```python
from build123d import *

# Parameters (mm, degrees)
F0_R     = 5
F1_DEPTH = 20
F2_R     = 1.25
F3_DEPTH = 20.001
F5_DEPTH = 10


with BuildPart() as f1:
    # F0 (on Front) → F1 (new body)
    with BuildSketch(Plane.XZ):
        Circle(F0_R)
    extrude(amount=F1_DEPTH)

    # F2 (on face) → F3 (cut, through all)
    with BuildSketch(Plane(origin=(0, 0, 0), x_dir=(-1, 0, 0), z_dir=(0, 1, 0))):
        Circle(F2_R)
    extrude(amount=-F3_DEPTH, mode=Mode.SUBTRACT)

    # F4 (on Front) → F5 (cut)
    with BuildSketch(Plane.XZ):
        Polygon((1.674316, 2.9), (-1.674316, 2.9), (-3.348632, 0), (-1.674316, -2.9), (1.674316, -2.9), (3.348632, 0), align=None)
    extrude(amount=F5_DEPTH, mode=Mode.SUBTRACT)


solid = f1.part
```
Can you work these out from the model? Positions are in its coordinate system, mm. A direction names the side the tool comes from. Round coordinates to 2 decimals unless told otherwise and drop trailing zeros. Loops run counter-clockwise (first coordinate to the right, second up) from the corner with the lowest first, then second, coordinate; pieces in that order, holes last.
Item 1: Suppose I cut it at B-B, the plane y = -8.75. Write out the boundary of the cut face in (x, z), then the cut area to 3 significant figures.
Item 2: Will these pins go through, and if not, where does the flat tip stop? pin 1 Ø1.5 at (x, y) = (-1.5, -3.5) entering from +Z; pin 2 Ø1 at (x, z) = (1.5, 0.5) entering from +Y; pin 3 Ø1 at (y, z) = (-2.5, -4) entering from +X.
Item 3: Please list where these lines run through material, in increasing order: L1, parallel to Z at x = 0, y = -15.5; L2, parallel to Y at x = 1, z = -2.25; L3, parallel to Z at x = 1.25, y = -9.
Item 4: Suppose I cut it at C-C, the plane z = -0.75. Write out the boundary of the cut face in (x, y).
Item 5: Which directions (+Z, -Z, +X, -X, +Y, -Y) give clear straight access to the entire face, cutting with the end or side of a thin tool? Please do faces 4 (the cylindrical face through (0.27, -14.93, -1.22)), 5 (the flat face through (2.5, -4.93, -1.47)).
Item 6: Suppose I cut it at A-A, the plane x = 0. Write out the boundary of the cut face in (y, z), then the cut area to 3 significant figures.
Item 7: Suppose I cut it at D-D, the plane x = -2. Write out the boundary of the cut face in (y, z), then the cut area to 3 significant figures.
Item 8: If we mould it in two halves opening along X, with no side actions, what happens to faces 1 (the cylindrical face through (-1.08, -9.86, -4.88)), 2 (the flat face through (1, -20, -1)), 3 (the flat face through (1.44, -10, 0.04))? For each: +X half, -X half, draft (parallel to the pull), parting line (faces both ways), or undercut.
Reported:
1. outline: circle Ø10 at (0, 0); hole (-3.35, 0) - (-1.67, -2.9) - (1.67, -2.9) - (3.35, 0) - (1.67, 2.9) - (-1.67, 2.9) - close
1. area: 49.4 mm2
2. pin 1: stops at z = 4.94
2. pin 2: stops at y = -10
2. pin 3: stops at x = 3.57
3. L1: z = -5 to -1.25, 1.25 to 5
3. L2: y = -20 to -10
3. L3: z = -4.84 to -2.9, 2.9 to 4.84
4. outline: (-4.94, -20) - (-1, -20) - (-1, -10) - (-2.92, -10) - (-2.92, 0) - (-4.94, 0) - close; (1, -20) - (4.94, -20) - (4.94, 0) - (2.92, 0) - (2.92, -10) - (1, -10) - close
5. face 4: +Y, -Y
5. face 5: +Y
6. outline: (-20, -5) - (0, -5) - (0, -2.9) - (-10, -2.9) - (-10, -1.25) - (-20, -1.25) - close; (-20, 1.25) - (-10, 1.25) - (-10, 2.9) - (0, 2.9) - (0, 5) - (-20, 5) - close
6. area: 117 mm2
7. outline: (-20, -4.58) - (0, -4.58) - (0, -2.34) - (-10, -2.34) - (-10, 2.34) - (0, 2.34) - (0, 4.58) - (-20, 4.58) - close
7. area: 137 mm2
8. face 1: parting line
8. face 2: draft
8. face 3: undercut
